Build history of the part. All positions in model axes, mm. Face numbers are marked on the shaded views. A direction names the side the tool comes from. Coordinates: 2 decimals unless noted, no trailing zeros. Loops run counter-clockwise (first coordinate to the right, second up) from the corner with the lowest first, then second, coordinate; pieces in that order, holes last.
(1) Slice it at A-A (y = 0). Give the cut face in (x, z), and give its area (4 significant figures).
(2) Flat gauge pins, fed straight in: P1, Ø1.8, axis at x = -1, y = 1.5, coming from the +Z side; P2, Ø3, axis at x = 3.5, z = -2, coming from the +Y side; P3, Ø6, axis at x = -2.5, z = -1.5, coming from the -Y side. Where does each tip first touch, or does it go through?
(3) Wall check: L1, parallel to Y at x = -3.75, z = 0; L2, parallel to Z at x = -0.75, y = 2.75; L3, parallel to Z at x = 2.5, y = 0.8. Give the ranges that are in metal, low to high.
(4) Two-plate mould, pull along Z, no slides. Class the marked faces 1, 2 and 3: pulls with the +Z half, pulls with the -Z half, needs draft (parallel to the pull), parting line crosses it, or undercut.
(5) Slice it at D-D (x = 1.25). Give the cut face in (y, z).
(6) Slice it at C-C (z = -9). Give the cut face in (x, y).
(7) Slice it at B-B (x = -0.75). Give the cut face in (y, z), and give its area (3 significant figures).
(8) Tool access for the marked faces 4, 5 and 6: list every direction of +Z, -Z, +X, -X, +Y, -Y with a clear straight run to the whole face (end or side of a thin tool).
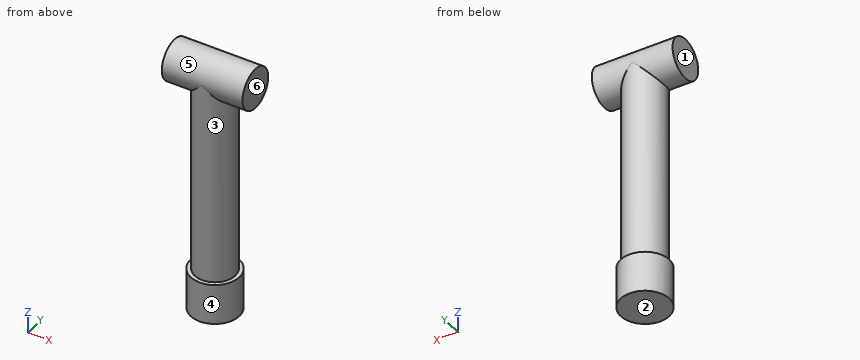
from build123d import *

# Parameters (mm, degrees)
SKETCH1_R                = 2.5
BOSS_EXTRUDE1_DEPTH      = 30
BOSS_EXTRUDE2_DEPTH      = 5
BOSS_EXTRUDE2_DEPTH_BACK = 5
SKETCH2_R                = 2.5
SKETCH3_R                = 3
BOSS_EXTRUDE3_DEPTH      = 5


with BuildPart() as part:
    # Sketch1 → Boss-Extrude1 (new body)
    with BuildSketch(Plane.XY):
        Circle(SKETCH1_R)
    extrude(amount=-BOSS_EXTRUDE1_DEPTH)

    # Sketch2 → Boss-Extrude2 (add, two sides: drawn at the far end of the back side and taken through both)
    with BuildSketch(Plane(origin=(0, 0, 0), x_dir=(0, 0, -1), z_dir=(1, 0, 0)).offset(-BOSS_EXTRUDE2_DEPTH_BACK)):
        Circle(SKETCH2_R)
    extrude(amount=BOSS_EXTRUDE2_DEPTH + BOSS_EXTRUDE2_DEPTH_BACK)

    # Sketch3 → Boss-Extrude3 (add)
    with BuildSketch(Plane(origin=(0, 0, -30), x_dir=(-1, 0, 0), z_dir=(0, 0, -1))):
        Circle(SKETCH3_R)
    extrude(amount=-BOSS_EXTRUDE3_DEPTH)


solid = part.part
Response values:
1. outline: (-5, -2.5) - (-2.5, -2.5) - (-2.5, -25) - (-3, -25) - (-3, -30) - (3, -30) - (3, -25) - (2.5, -25) - (2.5, -2.5) - (5, -2.5) - (5, 2.5) - (-5, 2.5) - close
1. area: 192.5 mm2
2. P1: stops at z = 2.43
2. P2: stops at y = 2.45
2. P3: stops at y = -2.5
3. L1: y = -2.5 to 2.5
3. L2: z = -30 to -25
3. L3: z = -30 to -25, -2.37 to 2.37
4. face 1: needs draft
4. face 2: pulls with the -Z half
4. face 3: undercut
5. outline: (-2.73, -30) - (2.73, -30) - (2.73, -25) - (2.17, -25) - (2.17, -1.25) arc R2.5 ccw (long way) to (-2.17, -1.25) - (-2.17, -25) - (-2.73, -25) - close
6. outline: circle Ø5 at (0, 0)
7. outline: (-2.9, -30) - (2.9, -30) - (2.9, -25) - (2.38, -25) - (2.38, -0.75) arc R2.5 ccw (long way) to (-2.38, -0.75) - (-2.38, -25) - (-2.9, -25) - close
7. area: 158 mm2
8. face 4: -Z
8. face 5: none
8. face 6: +Z, -Z, +X, +Y, -Y
